The model under review builds one solid part; all positions refer to its coordinate system, in mm. Face numbers are marked on the shaded views. A direction names the side the tool comes from. Coordinates: 2 decimals unless noted, no trailing zeros. Loops run counter-clockwise (first coordinate to the right, second up) from the corner with the lowest first, then second, coordinate; pieces in that order, holes last. Notation, with made-up numbers: M -2,11 L 11,11 A17 cw 11,32 Z; hole C 46,84.25 d5. An arc over 180 degrees is marked long. Return JSON: item names as keys, results as strings.
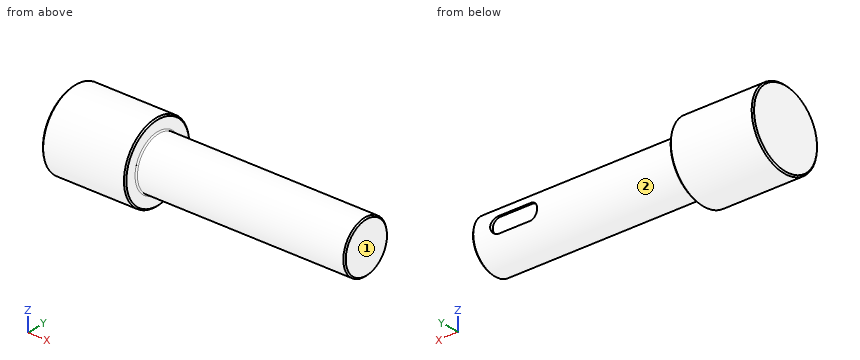
```python
from build123d import *

# Parameters (mm, degrees)
CHAMFER_1_SIZE      = 0.5
FILLET_1_R          = 0.5
CUT_EXTRUDE_1_DEPTH = 1.2


with BuildPart() as part:
    # Эскиз1 → Повернуть1 (revolve)
    with BuildSketch(Plane.XY):
        Polygon((0, 0), (0, 15), (32, 15), (32, 10), (112, 10), (112, 0), align=None)
    revolve(axis=Axis((112, 0, 0), (-1, 0, 0)))

    # Фаска1
    chamfer_1_edges = [part.edges().sort_by_distance(p)[0] for p in [
        (112, -10, 0),
        (32, -15, 0),
        (0, -15, 0),
    ]]
    chamfer(chamfer_1_edges, length=CHAMFER_1_SIZE)

    # Скругление1
    fillet_1_edges = [part.edges().sort_by_distance(p)[0] for p in [
        (32, -10, 0),
    ]]
    fillet(fillet_1_edges, radius=FILLET_1_R)

    # Эскиз2 → Вырез-Вытянуть1 (cut)
    with BuildSketch(Plane(origin=(0, 10, 0), x_dir=(1, 0, 0), z_dir=(0, 1, 0))):
        with BuildLine():
            Line((90, 3), (102, 3))
            ThreePointArc((102, 3), (105, 0), (102, -3))
            Line((102, -3), (90, -3))
            ThreePointArc((90, -3), (87, 0), (90, 3))
        make_face()
    extrude(amount=-CUT_EXTRUDE_1_DEPTH, mode=Mode.SUBTRACT)


solid = part.part
```
1. Machinability: for the marked faces 1 and 2, which of the approach directions +Z, -Z, +X, -X, +Y, -Y give a long, thin tool a straight path to every point of the face, cutting with its end or side? Answer none if there is none.
Check values:
{"face 1": "+Z, -Z, +X, +Y, -Y", "face 2": "+X"}
2. Insertion check: pin 1 Ø5 at (x, z) = (96.5, 0) entering from +Y; pin 2 Ø5 at (x, y) = (26.5, -9.5) entering from -Z; pin 3 Ø5 at (x, z) = (61, 10.5) entering from -Y. Each pin has a flat end and moves straight along its axis. Give the tip position at first contact, or say it passes through.
Check values:
{"pin 1": "y = 8.8", "pin 2": "z = -13.27", "pin 3": "y = -6"}
3. Add section C-C on x = 29. Give the boundary of the cut face in (y, z).
Check values:
{"outline": "C 0,0 d30"}
4. To check wall thickness, follow line 1 (X direction, y = 11.25, z = 0.5); line 2 (Y direction, x = 93, z = 1.5); line 3 (Z direction, x = 60, y = -8). State the ranges of each line that lie inside material, in increasing order.
Check values:
{"line 1": "0 to 32", "line 2": "-9.89 to 8.8", "line 3": "-6 to 6"}
5. Add section A-A on y = 0. Give the boundary of the cut face in (x, z), plus the area to 3 significant figures.
Check values:
{"outline": "M 0,-14.5 L 0.5,-15 L 31.5,-15 L 32,-14.5 L 32,-10.5 A0.5 cw 32.5,-10 L 111.5,-10 L 112,-9.5 L 112,9.5 L 111.5,10 L 32.5,10 A0.5 cw 32,10.5 L 32,14.5 L 31.5,15 L 0.5,15 L 0,14.5 Z", "area": "2,560 mm²"}
6. Add section B-B on z = 0. Give the boundary of the cut face in (x, y).
Check values:
{"outline": "M 0,-14.5 L 0.5,-15 L 31.5,-15 L 32,-14.5 L 32,-10.5 A0.5 cw 32.5,-10 L 111.5,-10 L 112,-9.5 L 112,9.5 L 111.5,10 L 105,10 L 105,8.8 L 87,8.8 L 87,10 L 32.5,10 A0.5 cw 32,10.5 L 32,14.5 L 31.5,15 L 0.5,15 L 0,14.5 Z"}
